Part print with two shaded views. Sizes in mm from the minimum x, y, z corner. A direction names the side the tool comes from. Round coordinates to 2 decimals unless told otherwise and drop trailing zeros. Loops run counter-clockwise (first coordinate to the right, second up) from the corner with the lowest first, then second, coordinate; pieces in that order, holes last.
(1) Flat gauge pins, fed straight in: pin 1 (6 mm diameter, centred on x = 94, y = 31, fed in from -Z); pin 2 (1.5 mm diameter, centred on x = 11, z = 1.5, fed in from +Y); pin 3 (1.5 mm diameter, centred on y = 179.5, z = 3, fed in from -X); pin 4 (4 mm diameter, centred on y = 6, z = 2.5, fed in from +X). Where does each tip first touch, or does it go through?
(2) Cut at B-B on x = 16. List the corners of the cut face in (y, z).
(3) Cut at A-A on z = 2.75. List the corners of the cut face in (x, y), then the cut area to 3 significant figures.
(4) Probe probe 1 along X at (y, z) = (175.5, 0.75). List the from-to ranges inside material, lowest first.
(5) Tool access for the marked faces 1 and 2: list every direction of +Z, -Z, +X, -X, +Y, -Y with a clear straight run to the whole face (end or side of a thin tool).
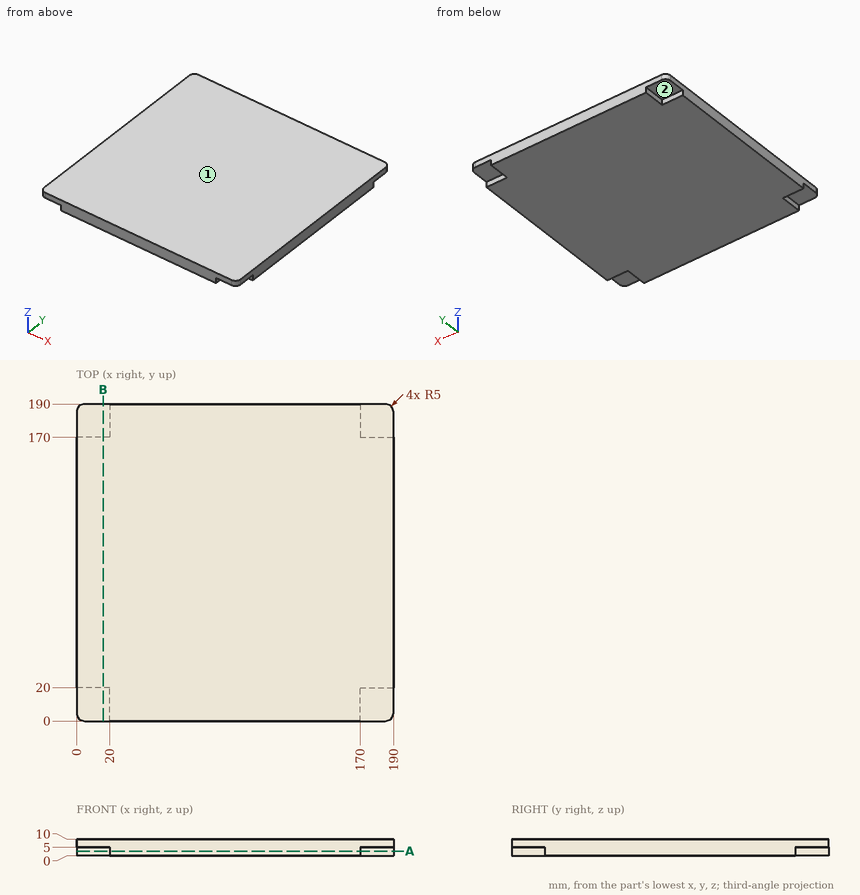
Final values:
1. pin 1: stops at z = 0
1. pin 2: stops at y = 170
1. pin 3: stops at x = 20
1. pin 4: stops at x = 170
2. outline: (0, 5) - (20, 5) - (20, 0) - (170, 0) - (170, 5) - (190, 5) - (190, 10) - (0, 10) - close
3. outline: (0, 20) - (20, 20) - (20, 0) - (170, 0) - (170, 20) - (190, 20) - (190, 170) - (170, 170) - (170, 190) - (20, 190) - (20, 170) - (0, 170) - close
3. area: 34,500 mm2
4. probe 1: x = 20 to 170
5. face 1: +Z, +X, -X, +Y, -Y
5. face 2: -Z, -X, +Y
